```python
from build123d import *

# Parameters (mm, degrees)
BOSS_EXTRUDE1_DEPTH       = 3.18
SKETCH2_4_OUTSIDE_W       = 40.858
SKETCH2_4_OUTSIDE_H       = 68.888
SKETCH2_4_OUTSIDE_R       = 5
CUT_EXTRUDE2_DEPTH        = 3.18
FILLET6_R                 = 3
M2X0_4_TAPPED_HOLE1_D     = 1.6
M2X0_4_TAPPED_HOLE1_DEPTH = 5.519311505
M2X0_4_TAPPED_HOLE1_TIP   = 0.480688495
SKETCH10_W                = 10
SKETCH10_H                = 10
CUT_EXTRUDE4_DEPTH        = 10


with BuildPart() as part:
    # Sketch2 → Boss-Extrude1 (new body)
    with BuildSketch(Plane(origin=(0, 0, 0), x_dir=(0, 0, -1), z_dir=(1, 0, 0))):
        Polygon((-7.39959254, 19.413571875), (10.60040746, 19.413571875), (10.60040746, -3.586428125), (4.27040746, -9.916428125), (4.27040746, -21.406428125), (10.625315102, -22.406428125), (17.27040746, -21.406428125), (17.27040746, -24.406428125), (2.77040746, -24.406428125), (2.77040746, -35.286428125), (-7.39959254, -35.286428125), (-7.39959254, -17.586428125), (-9.39959254, -15.586428125), (-9.39959254, -5.586428125), (-7.39959254, -3.586428125), align=None)
    extrude(amount=-BOSS_EXTRUDE1_DEPTH)

    # Sketch2<4> outside → Cut-Extrude2 (cut)
    # profile 1 of 3: a face of its own
    with BuildSketch(Plane(origin=(0, 0, 0), x_dir=(0, 0, -1), z_dir=(1, 0, 0))):
        with Locations((3.935, -7.936)):
            Rectangle(SKETCH2_4_OUTSIDE_W, SKETCH2_4_OUTSIDE_H)
        Polygon((-7.39959254, 19.413571875), (10.60040746, 19.413571875), (10.60040746, -3.586428125), (4.27040746, -9.916428125), (4.27040746, -21.406428125), (10.625315102, -22.406428125), (17.27040746, -21.406428125), (17.27040746, -24.406428125), (2.77040746, -24.406428125), (2.77040746, -35.286428125), (-7.39959254, -35.286428125), (-7.39959254, -17.586428125), (-9.39959254, -15.586428125), (-9.39959254, -5.586428125), (-7.39959254, -3.586428125), align=None, mode=Mode.SUBTRACT)
    # profile 2 of 3: a face of its own
    with BuildSketch(Plane(origin=(0, 0, 0), x_dir=(0, 0, -1), z_dir=(1, 0, 0))):
        with Locations((-2.39959254, -10.586428125)):
            Circle(SKETCH2_4_OUTSIDE_R)
    # profile 3 of 3: a face of its own
    with BuildSketch(Plane(origin=(0, 0, 0), x_dir=(0, 0, -1), z_dir=(1, 0, 0))):
        with Locations((1.60040746, 5.524437773)):
            Circle(SKETCH2_4_OUTSIDE_R)
    extrude(amount=-CUT_EXTRUDE2_DEPTH, mode=Mode.SUBTRACT)

    # Fillet6
    fillet6_edges = [part.edges().sort_by_distance(p)[0] for p in [
        (-1.59, -3.586428125, 7.39959254),
        (-1.59, -5.586428125, 9.39959254),
        (-1.59, -15.586428125, 9.39959254),
        (-1.59, -17.586428125, 7.39959254),
        (-1.59, -35.286428125, 7.39959254),
        (-1.59, -9.916428125, -4.27040746),
        (-1.59, -3.586428125, -10.60040746),
    ]]
    fillet(fillet6_edges, radius=FILLET6_R)

    # M2x0.4 Tapped Hole1
    with Locations(Plane(origin=(0, 19.413571875, 0), x_dir=(1, 0, 0), z_dir=(0, 1, 0))):
        with Locations((-1.59, 8.10040746), (-1.59, -4.89959254)):
            Hole(M2X0_4_TAPPED_HOLE1_D / 2, depth=M2X0_4_TAPPED_HOLE1_DEPTH)
            with Locations((0, 0, -(M2X0_4_TAPPED_HOLE1_DEPTH + M2X0_4_TAPPED_HOLE1_TIP / 2))):  # 118° drill point
                Cone(0, M2X0_4_TAPPED_HOLE1_D / 2, M2X0_4_TAPPED_HOLE1_TIP, mode=Mode.SUBTRACT)


with BuildPart() as body_2:
    # Mirror1: mirrored copy
    add(part.part.mirror(Plane.ZY))

    # Sketch10 → Cut-Extrude4 (cut)
    with BuildSketch(Plane(origin=(3.18, 0, 0), x_dir=(0, 0, -1), z_dir=(1, 0, 0))):
        with Locations((1.60040746, 5.524437773)):
            Rectangle(SKETCH10_W, SKETCH10_H)
    extrude(amount=-CUT_EXTRUDE4_DEPTH, mode=Mode.SUBTRACT)


solid = body_2.part
```
Here's how the part is built. I have some questions about the finished solid (model axes, mm). A direction names the side the tool comes from. Round coordinates to 2 decimals unless told otherwise and drop trailing zeros. Write each loop counter-clockwise with the first axis right and the second up, starting at its lowest first coordinate (ties: lowest second). Pieces come first, ordered by that corner, then holes.
Q1. If we mould it in two halves opening along Z, with no side actions, what happens to faces 1 (the flat face through (2, 0.524, -2)), 2 (the flat face through (2, -23, -17.27)), 3 (the flat face through (2, 5, 3.4)), 4 (the flat face through (3.18, -1, -1))? For each: +Z half, -Z half, draft (parallel to the pull), parting line (faces both ways), or undercut.
Q2. Which directions (+Z, -Z, +X, -X, +Y, -Y) give clear straight access to the entire face, cutting with the end or side of a thin tool? Please do faces 5 (the cylindrical face through (1.486, 16.615, -8.894)), 6 (the flat face through (1.568, -21.913, -13.901)), 7 (the flat face through (2, -30, -2.77)), 8 (the flat face through (1.568, -6.719, -7.467)).
Q3. Will these pins go through, and if not, where does the flat tip stop? P1, Ø1.3, axis at x = 1.59, z = -8.1, coming from the -Y side; P2, Ø1, axis at x = 2, y = 8.5, coming from the +Z side; P3, Ø1, axis at x = 2, y = -29, coming from the -Z side.
Q4. Please list where these lines run through material, in increasing order: probe 1 along Z at (x, y) = (1.59, 16.55); probe 2 along Y at (x, z) = (0.85, -3.5); probe 3 along Z at (x, y) = (1.4, 5).
Q5. If we section it at A-A on y = 6.5: Write out the boundary of the cut face in (x, z).
Q6. If we section it at B-B on y = -31.5: Write out the boundary of the cut face in (x, z).
Q7. If we section it at C-C on y = -18: Write out the boundary of the cut face in (x, z).
Answer below:
1. face 1: undercut
1. face 2: -Z half
1. face 3: undercut
1. face 4: draft
2. face 5: +Y
2. face 6: +X, -X, +Y
2. face 7: -Z, +X, -X, -Y
2. face 8: -Z, +X, -X
3. P1: stops at y = -24.41
3. P2: stops at z = 7.4
3. P3: stops at z = -2.77
4. probe 1: z = -10.6 to -8.9, -7.3 to 4.1, 5.7 to 7.4
4. probe 2: y = -24.41 to 0.52, 10.52 to 19.41
4. probe 3: z = -10.6 to -6.6, 3.4 to 7.4
5. outline: (0, -10.6) - (3.18, -10.6) - (3.18, -6.6) - (0, -6.6) - close; (0, 3.4) - (3.18, 3.4) - (3.18, 7.4) - (0, 7.4) - close
6. outline: (0, -2.77) - (3.18, -2.77) - (3.18, 7.4) - (0, 7.4) - close
7. outline: (0, -4.27) - (3.18, -4.27) - (3.18, 7.52) - (0, 7.52) - close
